Verification items for the finished model (mm, model axes). A direction names the side the tool comes from. Round coordinates to 2 decimals unless told otherwise and drop trailing zeros. Order: outer loops, then holes, each group sorted by start corner. A loop starts at its lowest first (then second) coordinate and runs counter-clockwise, first axis right, second up. Notation, with made-up numbers: (34.5, -28) -> (55.5, -28) arc R28 ccw to (55.5, -1) -> close; hole circle Ø5 at (60, 86). An arc over 180 degrees is marked (long way). Write item = value, one per line. Start each with the question number.
Autodesk Inventor part; units mm, degrees
ref_plane "YZ Plane" through (0, 0, 0) normal (1, 0, 0) x (0, 1, 0)
ref_plane "XZ Plane" through (0, 0, 0) normal (0, 1, 0) x (-1, 0, 0)
ref_plane "XY Plane" through (0, 0, 0) normal (0, 0, 1) x (1, 0, 0)
sketch "Sketch1" plane through (0, 0, 0) normal (0, 0, 1) x (1, 0, 0)
  line L0 (0, 0) -> (20, 0)
  line L1 (20, 0) -> (20, 25)
  line L2 (0, 25) -> (0, 0)
  line L3 (0, 27.5) -> (-0.5738, 27.5)
  line L4 (20, 27.5) -> (20.5842, 27.5)
  arc A0 (-0.5738, 27.5) -> (0, 25) centre (7.6984, 28.0827) ccw
  arc A1 (20, 25) -> (20.5842, 27.5) centre (12.3264, 28.1114) ccw
  line L5 (-0.5738, 27.5) -> (20, 27.5)
  dimension "d0" = 20
  dimension "d1" = 25
extrude "Extrusion1" add sketch "Sketch1" along normal blind 12
fillet "Fillet1" radius 1.27 12 edges at (10, 0, 12) (20, 12.5, 12) (20, 0, 6) (20, 12.5, 0) (10, 0, 0) (0, 0, 6) (0, 12.5, 0) (0, 12.5, 12) (20.3896, 26.2272, 12) (20.3896, 26.2272, 0) (-0.3841, 26.2277, 0) (-0.3841, 26.2277, 12)
fillet "Fillet2" radius 0.127 7 edges at (-0.2004, 27.5, 11.6285) (-0.5738, 27.5, 6) (-0.2004, 27.5, 0.3715) (19.6696, 27.5, 0.0516) (20.5842, 27.5, 6) (19.6696, 27.5, 11.9484) (10.005, 27.5, 12)
sketch "Sketch2" plane through (1.27, 0, 1.27) normal (0, -1, 0) x (1, 0, 0)
  line L0 (0, 0) -> (-1.27, 0)
  line L1 (0, 9.46) -> (0, 10.73)
  line L2 (0, 0) -> (0, 9.46)
  circle A0 centre (8.73, 4.73) radius 1.5875
  point P0 (-1.27, -1.27)
extrude "Extrusion2" cut sketch "Sketch2" against normal blind 1.27
properties part number "Tc-1"
(1) Draft check along X on faces 1 (the flat face through (10, 27.5, 6)), 2 (the cylindrical face through (20.38, 26.18, 5.93)), 3 (the flat face through (10, 1.27, 6)), 4 (the cylindrical face through (8.414, 0.626, 6.07)). Enter one of: +X half, -X half, draft (parallel to the pull), parting line (faces both ways), or undercut.
(2) Depth check by flat-ended pin: pin 1 (1.5 mm diameter, centred on y = 22.5, z = 5, fed in from +X); pin 2 (4.5 mm diameter, centred on y = 8.5, z = 8, fed in from -X); pin 3 (1 mm diameter, centred on x = 17.5, z = 2.5, fed in from -Y); pin 4 (1 mm diameter, centred on x = 10, z = 5.5, fed in from -Y). Enter the tip coordinate at first touch or a pass-through.
(3) Cross-section at C-C (z = 6). Enter the section's corners in (x, y), and give its area (3 significant figures).
(4) Cross-section at A-A (z = 3.25). Enter the section's corners in (x, y).
(5) Scan lines: line 1 along Z through (x, y) = (10, 0.7); line 2 along Z through (x, y) = (10, 0.3); line 3 along X through (y, z) = (22, 9.75). Record each from-to range of solid material in increasing order. Write a range as from..to.
(6) Cross-section at B-B (y = 22.5). Enter the section's corners in (x, z).
(7) Set-up check for faces 5 (the cylindrical face through (19.618, 13.432, 11.638)), 6 (the cylindrical face through (19.638, 13.432, 0.382)), 7 (the flat face through (20, 13, 6)), 8 (the cylindrical face through (0.382, 13.095, 11.638)), 9 (the flat face through (0, 13, 6)): record each of +Z, -Z, +X, -X, +Y, -Y from which the full face is reachable in a straight line by a thin tool's end or side.
Outcome:
q1.face_1 = draft
q1.face_2 = +X half
q1.face_3 = undercut
q1.face_4 = undercut
q2.pin_1 = 20
q2.pin_2 = 0
q2.pin_3 = 0
q2.pin_4 = 1.27
q3.outline = (-0.56, 27.36) arc R8.29 ccw to (0, 25) -> (0, 1.27) arc R1.27 ccw to (1.27, 0) -> (8.41, 0) -> (8.41, 1.27) -> (11.59, 1.27) -> (11.59, 0) -> (18.73, 0) arc R1.27 ccw to (20, 1.27) -> (20, 25) arc R8.28 ccw to (20.57, 27.36) arc R0.13 ccw to (20.45, 27.5) -> (-0.44, 27.5) arc R0.13 ccw to start
q3.area = 547 mm^2
q4.outline = (-0.56, 27.36) arc R8.29 ccw to (0, 25) -> (0, 1.27) arc R1.27 ccw to (1.27, 0) -> (18.73, 0) arc R1.27 ccw to (20, 1.27) -> (20, 25) arc R8.28 ccw to (20.57, 27.36) arc R0.13 ccw to (20.45, 27.5) -> (-0.44, 27.5) arc R0.13 ccw to start
q5.line_1 = 0.14..4.41, 7.59..11.86
q5.line_2 = 0.45..4.41, 7.59..11.55
q5.line_3 = 0..20
q6.outline = (0, 1.27) arc R1.27 ccw to (1.27, 0) -> (18.73, 0) arc R1.27 ccw to (20, 1.27) -> (20, 10.73) arc R1.27 ccw to (18.73, 12) -> (1.27, 12) arc R1.27 ccw to (0, 10.73) -> close
q7.face_5 = +Z, +X, -Y
q7.face_6 = -Z, +X, -Y
q7.face_7 = +Z, -Z, +X, -Y
q7.face_8 = +Z, -X, -Y
q7.face_9 = +Z, -Z, -X, -Y
